```python
from build123d import *

# Parameters (mm, degrees)
SKETCH1_W           = 7.9
SKETCH1_H           = 10
BOSS_EXTRUDE1_DEPTH = 2.5
FILLET2_R           = 2
FILLET3_R           = 2
SKETCH4_R           = 1
CUT_EXTRUDE1_DEPTH  = 10
SKETCH5_R           = 1.5
BOSS_EXTRUDE2_DEPTH = 600


with BuildPart() as part:
    # Sketch1 → Boss-Extrude1 (new, symmetric)
    with BuildSketch(Plane.XY):
        Rectangle(SKETCH1_W, SKETCH1_H)
    extrude(amount=BOSS_EXTRUDE1_DEPTH, both=True)

    # Fillet2
    fillet2_edges = [part.edges().sort_by_distance(p)[0] for p in [
        (0, 5, -2.5),
    ]]
    fillet(fillet2_edges, radius=FILLET2_R)

    # Fillet3
    fillet3_edges = [part.edges().sort_by_distance(p)[0] for p in [
        (0, 5, 2.5),
    ]]
    fillet(fillet3_edges, radius=FILLET3_R)

    # Sketch4 → Cut-Extrude1 (cut)
    with BuildSketch(Plane(origin=(3.95, 0, 0), x_dir=(0, 0, -1), z_dir=(1, 0, 0))):
        with Locations(Location((0, 2.5, 0), (0, 0, 90))):
            Circle(SKETCH4_R)
    extrude(amount=-CUT_EXTRUDE1_DEPTH, mode=Mode.SUBTRACT)

    # Sketch5 → Boss-Extrude2 (add)
    with BuildSketch(Plane.XZ.offset(5)):
        with Locations(Location((0, 0, 0), (0, 0, 90))):
            Circle(SKETCH5_R)
    extrude(amount=BOSS_EXTRUDE2_DEPTH)


solid = part.part
```
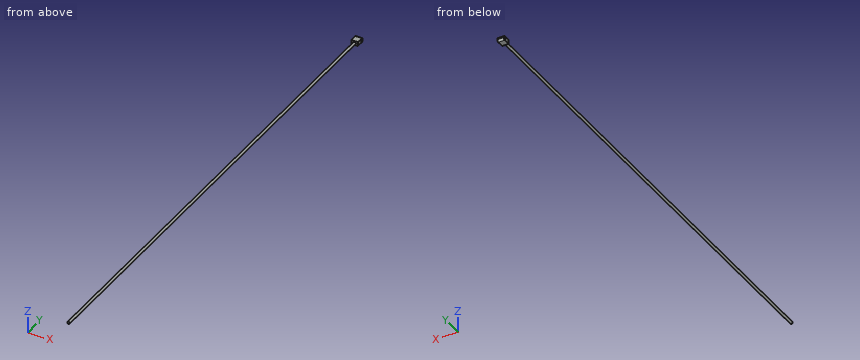
For this review, take the finished solid that the model builds, in its own axes (mm). Coordinates: 2 decimals unless noted, no trailing zeros. Write each loop counter-clockwise with the first axis right and the second up, starting at its lowest first coordinate (ties: lowest second). Pieces come first, ordered by that corner, then holes. Notation, with made-up numbers: (-11.5, 34) - (38.5, 34) arc R15 cw to (38.5, 50) - close; hole circle Ø5 at (-15.5, -32.5). An arc over 180 degrees is marked (long way). Answer in a Markdown table with one row per item. Add a question column.
Q1. We need section B-B, the plane y = -159.5. State the section outline as (x, z) points.
Q2. For probe 1 along Z at (x, y) = (1.25, 2.5); probe 2 along Y at (x, z) = (-1, 0.35); probe 3 along X at (y, z) = (-214, 0.15), list the stretches that pass through material, from the lowest coordinate up.
Q3. We need section A-A, the plane x = -2.75. State the section outline as (y, z) points, and give its area (3 significant figures).
Q4. For P1, Ø3, axis at y = -58.5, z = -1.5, coming from the -X side; P2, Ø4, axis at x = -1.5, y = -314, coming from the +Z side; P3, Ø1, axis at y = -252, z = 0, coming from the +X side; P4, Ø3, axis at y = 2.5, z = 0, coming from the -X side, all flat-tipped, find the tip position at first contact; note any pin that passes through.
Answer list:
| question | item | result |
|---|---|---|
| 1 | outline | circle Ø3 at (0, 0) |
| 2 | probe 1 | z = -2.5 to -1, 1 to 2.5 |
| 2 | probe 2 | y = -605 to 1.56, 3.44 to 5 |
| 2 | probe 3 | x = -1.49 to 1.49 |
| 3 | outline | (-5, -2.5) - (3, -2.5) arc R2 ccw to (5, -0.5) - (5, 0.5) arc R2 ccw to (3, 2.5) - (-5, 2.5) - close; hole circle Ø2 at (2.5, 0) |
| 3 | area | 45.1 mm2 |
| 4 | P1 | stops at x = -1.5 |
| 4 | P2 | stops at z = 1.5 |
| 4 | P3 | stops at x = 1.5 |
| 4 | P4 | stops at x = -3.95 |
